from build123d import *

# Parameters (mm, degrees)
SKETCH2_R           = 5
BOSS_EXTRUDE1_DEPTH = 10


with BuildPart() as part:
    # Sketch2 → Boss-Extrude1 (new, symmetric)
    with BuildSketch(Plane.XY):
        with BuildLine():
            ThreePointArc((85.88315603, 117.410181971), (70, 120), (54.11684397, 117.410181971))
            ThreePointArc((54.11684397, 117.410181971), (40, 121.961524227), (36.88315603, 107.4603076))
            ThreePointArc((36.88315603, 107.4603076), (26.698729811, 95), (21, 79.949874371))
            ThreePointArc((21, 79.949874371), (10, 70), (21, 60.050125629))
            ThreePointArc((21, 60.050125629), (26.698729811, 45), (36.88315603, 32.5396924))
            ThreePointArc((36.88315603, 32.5396924), (40, 18.038475773), (54.11684397, 22.589818029))
            ThreePointArc((54.11684397, 22.589818029), (70, 20), (85.88315603, 22.589818029))
            ThreePointArc((85.88315603, 22.589818029), (100, 18.038475773), (103.11684397, 32.5396924))
            ThreePointArc((103.11684397, 32.5396924), (113.301270189, 45), (119, 60.050125629))
            ThreePointArc((119, 60.050125629), (130, 70), (119, 79.949874371))
            ThreePointArc((119, 79.949874371), (113.301270189, 95), (103.11684397, 107.4603076))
            ThreePointArc((103.11684397, 107.4603076), (100, 121.961524227), (85.88315603, 117.410181971))
        make_face()
        with Locations((120, 70)):
            Circle(SKETCH2_R, mode=Mode.SUBTRACT)
        with Locations((95, 26.698729811)):
            Circle(SKETCH2_R, mode=Mode.SUBTRACT)
        with Locations((45, 26.698729811)):
            Circle(SKETCH2_R, mode=Mode.SUBTRACT)
        with Locations((20, 70)):
            Circle(SKETCH2_R, mode=Mode.SUBTRACT)
        with Locations((45, 113.301270189)):
            Circle(SKETCH2_R, mode=Mode.SUBTRACT)
        with Locations((95, 113.301270189)):
            Circle(SKETCH2_R, mode=Mode.SUBTRACT)
        with BuildLine():
            ThreePointArc((104.793766493, 90.088190451), (94.45783105, 101.874065989), (80.398412541, 108.80740392))
            ThreePointArc((80.398412541, 108.80740392), (74.058666579, 105.147149882), (77.718920616, 98.80740392))
            ThreePointArc((77.718920616, 98.80740392), (88.15546898, 93.660667831), (95.828011772, 84.911809549))
            ThreePointArc((95.828011772, 84.911809549), (102.899079583, 83.017122639), (104.793766493, 90.088190451))
        make_face(mode=Mode.SUBTRACT)
        with BuildLine():
            ThreePointArc((70, 29.823619098), (85.374835344, 32.881863994), (98.408991379, 41.591008621))
            ThreePointArc((98.408991379, 41.591008621), (98.408991379, 48.911516696), (91.088483304, 48.911516696))
            ThreePointArc((91.088483304, 48.911516696), (81.413004922, 42.44656873), (70, 40.176380902))
            ThreePointArc((70, 40.176380902), (64.823619098, 35), (70, 29.823619098))
        make_face(mode=Mode.SUBTRACT)
        with BuildLine():
            ThreePointArc((35.206233507, 90.088190451), (30.167333606, 75.244070016), (31.19259608, 59.601587459))
            ThreePointArc((31.19259608, 59.601587459), (37.532342042, 55.941333421), (41.19259608, 62.281079384))
            ThreePointArc((41.19259608, 62.281079384), (40.431526098, 73.892763439), (44.171988228, 84.911809549))
            ThreePointArc((44.171988228, 84.911809549), (42.277301319, 91.982877361), (35.206233507, 90.088190451))
        make_face(mode=Mode.SUBTRACT)
    extrude(amount=BOSS_EXTRUDE1_DEPTH, both=True)


solid = part.part
Build history of the part. All positions in model axes, mm. Round coordinates to 2 decimals unless told otherwise and drop trailing zeros. Order: outer loops, then holes, each group sorted by start corner. A loop starts at its lowest first (then second) coordinate and runs counter-clockwise, first axis right, second up. Notation, with made-up numbers: M -17,-4 L 38,-4 A23 cw 38,7 Z; hole C -17.75,28.5 d7. An arc over 180 degrees is marked long. Use CSV: the item, a comma, the result in double quotes. Start each with the question number.
(1) Cut at C-C on z = -2.25. State how many separate pieces and enclosed holes the cut face has, then the cut area to 3 significant figures.
(2) Cut at B-B on y = 105.5. List the corners of the cut face in (x, z).
(3) Cut at A-A on y = 70. List the corners of the cut face in (x, z), then the cut area to 3 significant figures.
(4) Flat gauge pins, fed straight in: P1, Ø8, axis at y = 60.5, z = -4, coming from the -X side; P2, Ø8, axis at x = 35.5, y = 77, coming from the -Z side; P3, Ø3, axis at x = 48.5, z = 1.5, coming from the +Y side; P4, Ø2, axis at x = 66.5, z = -2.5, coming from the +Y side. Where does each tip first touch, or does it go through?
(5) Drill centre lines: probe 1 along Y at (x, z) = (69.5, 8); probe 2 along X at (y, z) = (86.5, 1.75); probe 3 along X at (y, z) = (27, 8). Where is each one in solid material? Low to high.
(6) Mould opens along X. For faces 1 (the face through (69, 71, -10)), 2 (the face through (41.315, 116.681, -0.14)) say: +X half, -X half, draft (parallel to the pull), parting line (faces both ways), or undercut.
(7) Cut at D-D on y = 87.5. List the corners of the cut face in (x, z), then the cut area to 3 significant figures.
Findings:
1,separate pieces,"1"
1,enclosed holes,"9"
1,area,"7,260 mm^2"
2,outline,"M 34.79,-10 L 74.17,-10 L 74.17,10 L 34.79,10 Z; M 88.81,-10 L 105.21,-10 L 105.21,10 L 88.81,10 Z"
3,outline,"M 10,-10 L 15,-10 L 15,10 L 10,10 Z; M 25,-10 L 29.82,-10 L 29.82,10 L 25,10 Z; M 40.18,-10 L 115,-10 L 115,10 L 40.18,10 Z; M 125,-10 L 130,-10 L 130,10 L 125,10 Z"
3,area,"1,790 mm^2"
4,P1,"stops at x = 11.65"
4,P2,"passes through"
4,P3,"stops at y = 123.1"
4,P4,"stops at y = 119.94"
5,probe 1,"y = 20 to 29.85, 40.15 to 120"
5,probe 2,"x = 22.8 to 33.37, 44.77 to 94.84, 105.39 to 117.2"
5,probe 3,"x = 35 to 40.01, 49.99 to 90.01, 99.99 to 105"
6,face 1,"draft"
6,face 2,"undercut"
7,outline,"M 23.16,-10 L 33.84,-10 L 33.84,10 L 23.16,10 Z; M 44.87,-10 L 94.15,-10 L 94.15,10 L 44.87,10 Z; M 105.49,-10 L 116.84,-10 L 116.84,10 L 105.49,10 Z"
7,area,"1,430 mm^2"
